Verification items for the finished model (mm, model axes). A direction names the side the tool comes from. Coordinates: 2 decimals unless noted, no trailing zeros. Order: outer loops, then holes, each group sorted by start corner. A loop starts at its lowest first (then second) coordinate and runs counter-clockwise, first axis right, second up. Notation, with made-up numbers: (74, 17) -> (86, 17) arc R15 cw to (86, 43) -> close; hole circle Ø9 at (11, 29.25). An arc over 180 degrees is marked (long way). Answer as CSV lines item,"result".
```python
from build123d import *

# Parameters (mm, degrees)
SKETCH097_W              = 26
SKETCH097_H              = 46
PAD029_DEPTH             = 30
POCKET062_DEPTH          = 5
SKETCH099_W              = 20.25
SKETCH099_H              = 40.5
POCKET063_DEPTH          = 25
SKETCH100_R              = 1.6
PAD030_DEPTH             = 3
SKETCH101_W              = 8
SKETCH101_H              = 18.5
PAD031_DEPTH             = 30
POCKET064_DEPTH          = 46.001
SKETCH103_R              = 1.65
POCKET065_DEPTH          = 46.001
SKETCH104_R              = 1.65
POCKET066_DEPTH          = 26.001
CHAMFER009002001002_SIZE = 5
CHAMFER009002001003_SIZE = 5
CHAMFER009002001004_SIZE = 1
CHAMFER009002001005_SIZE = 0.4


with BuildPart() as part:
    # Sketch097 → Pad029 (new body)
    with BuildSketch(Plane.XY):
        with Locations((13, -3)):
            Rectangle(SKETCH097_W, SKETCH097_H)
    extrude(amount=PAD029_DEPTH)

    # Sketch098 (on Face5 of Pad029) → Pocket062 (cut)
    with BuildSketch(Plane(origin=(0, 0, 0), x_dir=(1, 0, 0), z_dir=(0, 0, -1))):
        with BuildLine():
            ThreePointArc((-6.067125, 20), (-14.778532, -14.778532), (20, -6.067125))
            Line((20, 6.067125), (20, -6.067125))
            ThreePointArc((20, 6.067125), (14.778532, 14.778532), (6.067125, 20))
            Line((-6.067125, 20), (6.067125, 20))
        make_face()
    extrude(amount=-POCKET062_DEPTH, mode=Mode.SUBTRACT)

    # Sketch099 (on Face6 of Pocket062) → Pocket063 (cut)
    with BuildSketch(Plane.XY.offset(30)):
        with Locations((10.125, 0)):
            Rectangle(SKETCH099_W, SKETCH099_H)
    extrude(amount=-POCKET063_DEPTH, mode=Mode.SUBTRACT)

    # Sketch100 (on Face7 of Pocket063) → Pad030 (join)
    with BuildSketch(Plane.XY.offset(5)):
        with Locations((16, 16)):
            Circle(SKETCH100_R)
        with Locations((16, -16)):
            Circle(SKETCH100_R)
    extrude(amount=PAD030_DEPTH)

    # Sketch101 (on Face5 of Pad030) → Pad031 (join)
    with BuildSketch(Plane.XY.offset(30)):
        with Locations((30, -16.75)):
            Rectangle(SKETCH101_W, SKETCH101_H)
    extrude(amount=-PAD031_DEPTH)

    # Sketch102 (on Face19 of Pad031) → Pocket064 (cut, through all)
    with BuildSketch(Plane.XZ.offset(26)):
        Polygon((34, 12), (26, 0), (34, 0), align=None)
        Polygon((34, 30), (26, 30), (34, 18), align=None)
    extrude(amount=-POCKET064_DEPTH, mode=Mode.SUBTRACT)

    # Sketch103 (on Face21 of Pocket064) → Pocket065 (cut, through all)
    with BuildSketch(Plane.XZ.offset(26)):
        with Locations((7, 23)):
            Circle(SKETCH103_R)
        with Locations((30, 15)):
            Circle(SKETCH103_R)
    extrude(amount=-POCKET065_DEPTH, mode=Mode.SUBTRACT)

    # Sketch104 (on Face4 of Pocket065) → Pocket066 (cut, through all)
    with BuildSketch(Plane.YZ.offset(26)):
        with Locations((13, 23)):
            Circle(SKETCH104_R)
    extrude(amount=-POCKET066_DEPTH, mode=Mode.SUBTRACT)

    # Chamfer009002001002
    chamfer009002001002_edges = [part.edges().sort_by_distance(p)[0] for p in [
        (0, -23.125, 30),
        (23.125, 20, 30),
        (0, -23, 0),
    ]]
    chamfer(chamfer009002001002_edges, length=CHAMFER009002001002_SIZE)

    # Chamfer009002001003
    chamfer009002001003_edges = [part.edges().sort_by_distance(p)[0] for p in [
        (6.067125, 20, 2.5),
    ]]
    chamfer(chamfer009002001003_edges, length=CHAMFER009002001003_SIZE)

    # Chamfer009002001004
    chamfer009002001004_edges = [part.edges().sort_by_distance(p)[0] for p in [
        (0, -26, 15),
        (2.5, -26, 2.5),
        (15.5, -26, 0),
        (30, -26, 6),
        (34, -26, 15),
        (30, -26, 24),
        (2.5, -26, 27.5),
        (15.5, -26, 30),
    ]]
    chamfer(chamfer009002001004_edges, length=CHAMFER009002001004_SIZE)

    # Chamfer009002001005
    chamfer009002001005_edges = [part.edges().sort_by_distance(p)[0] for p in [
        (5.35, -26, 23),
        (28.35, -26, 15),
        (28.35, -7.5, 15),
        (26, 11.35, 23),
        (14.4, 16, 8),
        (14.4, -16, 8),
        (5.35, -20.25, 23),
    ]]
    chamfer(chamfer009002001005_edges, length=CHAMFER009002001005_SIZE)


with BuildPart() as part_1:
    # Body011 placement: moved
    add(part.part.moved(Location((0, 0, -10))))


solid = part_1.part
```
Item 1: Section check B-B, the plane y = -21.5. Record the boundary of the cut face in (x, z), plus the area to 3 significant figures.
Answer list:
outline,"(0, -5) -> (5, -10) -> (26, -10) -> (34, 2) -> (34, 8) -> (26, 20) -> (5, 20) -> (0, 15) -> close; hole circle Ø3.3 at (7, 13); hole circle Ø3.3 at (30, 5)"
area,"882 mm2"
Item 2: Depth check by flat-ended pin: pin 1 Ø5 at (y, z) = (-20, -5) entering from +X; pin 2 Ø6 at (x, z) = (6.5, 9) entering from +Y; pin 3 Ø4 at (x, z) = (29, 5) entering from +Y. Enter the tip coordinate at first touch or a pass-through.
Answer list:
pin 1,"x = 31"
pin 2,"y = -20.25"
pin 3,"y = -7.5"
Item 3: Thickness scan on line 1 (Z direction, x = 23.7, y = 13); line 2 (Y direction, x = 18, z = 7.5); line 3 (X direction, y = 7, z = 14.5). Record the ranges inside material, lowest first.
Answer list:
line 1,"-10 to 11.35, 14.65 to 20"
line 2,"-26 to -20.25"
line 3,"20.25 to 26"
Item 4: Release check for a two-part mould opening along X. For faces 4 (the cylindrical face through (14.4, 16.07, -3.72)), 5 (the cylindrical face through (28.69, -16.87, 4)), 6 (the flat face through (23, 18, 17)), 7 (the flat face through (33.5, -25.5, 5)) record: +X half, -X half, draft (parallel to the pull), parting line (faces both ways), or undercut.
Answer list:
face 4,"undercut"
face 5,"undercut"
face 6,"draft"
face 7,"+X half"
Item 5: Section check C-C, the plane z = 5. Record the boundary of the cut face in (x, y), plus the area to 3 significant figures.
Answer list:
outline,"(0, -25) -> (1, -26) -> (27.95, -26) -> (28.35, -25.6) -> (28.35, -7.9) -> (27.95, -7.5) -> (26, -7.5) -> (26, 20) -> (20.25, 20) -> (20.25, -20.25) -> (0, -20.25) -> close; (31.65, -25.6) -> (32.05, -26) -> (33, -26) -> (34, -25) -> (34, -7.5) -> (32.05, -7.5) -> (31.65, -7.9) -> close"
area,"467 mm2"
Item 6: Tool access check on faces 1 (the flat face through (27, -7.5, 5)), 2 (the flat face through (34, -16, 5)), 3 (the flat face through (20, 0, -8)). Record the directions out of +Z, -Z, +X, -X, +Y, -Y that give a thin tool (end or side, any length) a straight path to the whole face; none if there is none.
Answer list:
face 1,"+Z, -Z, +X, +Y"
face 2,"+Z, -Z, +X, +Y, -Y"
face 3,"+Z, -Z, -X"
Item 7: Section check A-A, the plane x = 24. Record the boundary of the cut face in (y, z).
Answer list:
outline,"(-26, -9) -> (-25, -10) -> (20, -10) -> (20, 15) -> (15, 20) -> (-25, 20) -> (-26, 19) -> close; hole circle Ø3.3 at (13, 13)"
Item 8: Section check D-D, the plane x = 7. Record the boundary of the cut face in (y, z).
Answer list:
outline,"(-26, -9) -> (-25, -10) -> (-19.69, -10) -> (-19.69, -5) -> (-20.25, -5) -> (-20.25, 10.95) -> (-20.65, 11.35) -> (-25.6, 11.35) -> (-26, 10.95) -> close; (-26, 15.05) -> (-25.6, 14.65) -> (-20.65, 14.65) -> (-20.25, 15.05) -> (-20.25, 20) -> (-25, 20) -> (-26, 19) -> close"
